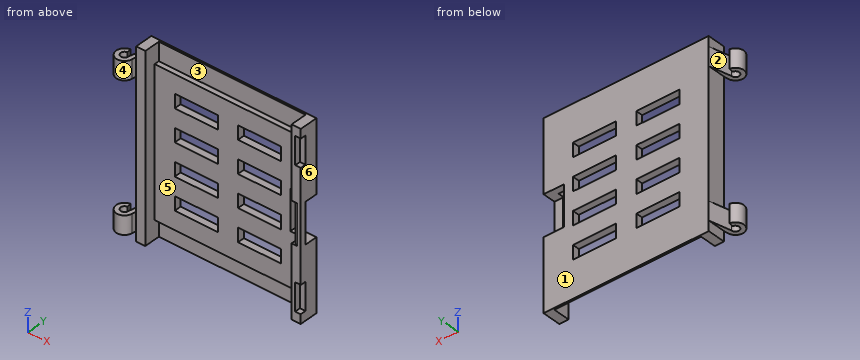
from build123d import *

# Parameters (mm, degrees)
SKETCH1_W           = 3.175
SKETCH1_H           = 1.27
SKETCH1_H_2         = 1.9685
BOSS_EXTRUDE1_DEPTH = 31.75
SKETCH1_4_W         = 3.175
SKETCH1_4_H         = 1.27
CUT_EXTRUDE1_DEPTH  = 6.985
SKETCH2_W           = 3.429
SKETCH2_H           = 10.222992
SKETCH2_W_2         = 13.9065
SKETCH2_W_3         = 6.35
CUT_EXTRUDE2_DEPTH  = 19.05
SKETCH4_W           = 14.9225
SKETCH4_H           = 4.7625
CUT_EXTRUDE4_DEPTH  = 3.38125
CUT_EXTRUDE7_DEPTH  = 6.985
SKETCH9_W           = 50.8
SKETCH9_H           = 1.74625
CUT_EXTRUDE8_DEPTH  = 6.35
SKETCH10_W          = 9.525
SKETCH10_H          = 1.905
CUT_EXTRUDE9_DEPTH  = 1.905
SKETCH11_W          = 3.175
SKETCH11_H          = 0.1905
CUT_EXTRUDE10_DEPTH = 64.5
FILLET2_R           = 0.127


with BuildPart() as part:
    # Sketch1 → Boss-Extrude1 (new body, symmetric)
    with BuildSketch(Plane.XY):
        Polygon((-28.575, 6.35), (-28.575, 0), (-25.4, 0), (-25.4, 3.96875), (21.59, 3.96875), (21.59, 6.35), align=None)
        with BuildLine():
            Line((-28.719147778, -1.313425633), (-28.575, 0))
            Line((-28.575, 0), (-28.575, 6.35))
            Line((-28.575, 6.35), (-30.257496, -0.999998))
            ThreePointArc((-30.257496, -0.999998), (-32.447762596, -1.986950865), (-31.736171426, 0.307603934))
            Line((-31.736171426, 0.307603934), (-31.926464573, 1.851416204))
            ThreePointArc((-31.926464573, 1.851416204), (-33.592921231, -3.045007588), (-28.719147778, -1.313425633))
        make_face()
        Polygon((28.575, 6.35), (21.59, 6.35), (21.59, 3.96875), (25.4, 3.96875), (25.4, 3.2385), (28.575, 3.2385), align=None)
        with Locations((26.9875, 2.6035)):
            Rectangle(SKETCH1_W, SKETCH1_H)
        with Locations((26.9875, 0.98425)):
            Rectangle(SKETCH1_W, SKETCH1_H_2)
    extrude(amount=BOSS_EXTRUDE1_DEPTH, both=True)

    # Sketch1_4 → Cut-Extrude1 (cut, symmetric)
    with BuildSketch(Plane.XY):
        with Locations((26.9875, 2.6035)):
            Rectangle(SKETCH1_4_W, SKETCH1_4_H)
        Polygon((28.575, 6.35), (21.59, 6.35), (21.59, 3.96875), (25.4, 3.96875), (25.4, 3.2385), (28.575, 3.2385), align=None)
    extrude(amount=CUT_EXTRUDE1_DEPTH, both=True, mode=Mode.SUBTRACT)

    # Sketch2 → Cut-Extrude2 (cut)
    with BuildSketch(Plane(origin=(-28.575, 9.604995709, 0), x_dir=(0, 0, 1), z_dir=(-1, 0, 0))):
        with Locations((-30.0355, -8.366491709)):
            Rectangle(SKETCH2_W, SKETCH2_H)
        with Locations((-15.01775, -8.366491709)):
            Rectangle(SKETCH2_W_2, SKETCH2_H)
        with Locations((-4.8895, -8.366491709)):
            Rectangle(SKETCH2_W_3, SKETCH2_H)
        with Locations((4.8895, -8.366491709)):
            Rectangle(SKETCH2_W_3, SKETCH2_H)
        with Locations((15.01775, -8.366491709)):
            Rectangle(SKETCH2_W_2, SKETCH2_H)
        with Locations((30.0355, -8.366491709)):
            Rectangle(SKETCH2_W, SKETCH2_H)
        with Locations((0, -8.366491709)):
            Rectangle(SKETCH2_W, SKETCH2_H)
    extrude(amount=CUT_EXTRUDE2_DEPTH, mode=Mode.SUBTRACT)

    # Sketch4 → Cut-Extrude4 (cut, through all)
    with BuildSketch(Plane.XZ.offset(-3.96875)):
        with Locations((-10.95375, 16.66875)):
            Rectangle(SKETCH4_W, SKETCH4_H)
        with Locations((10.95375, 16.66875)):
            Rectangle(SKETCH4_W, SKETCH4_H)
        with Locations((-10.95375, 5.55625)):
            Rectangle(SKETCH4_W, SKETCH4_H)
        with Locations((10.95375, 5.55625)):
            Rectangle(SKETCH4_W, SKETCH4_H)
        with Locations((-10.95375, -5.55625)):
            Rectangle(SKETCH4_W, SKETCH4_H)
        with Locations((10.95375, -5.55625)):
            Rectangle(SKETCH4_W, SKETCH4_H)
        with Locations((-10.95375, -16.66875)):
            Rectangle(SKETCH4_W, SKETCH4_H)
        with Locations((10.95375, -16.66875)):
            Rectangle(SKETCH4_W, SKETCH4_H)
    extrude(amount=-CUT_EXTRUDE4_DEPTH, mode=Mode.SUBTRACT)

    # Sketch8 → Cut-Extrude7 (cut, symmetric)
    with BuildSketch(Plane.XY):
        with BuildLine():
            ThreePointArc((27.432, 0), (26.172949082, 0.772949082), (25.4, 2.032))
            ThreePointArc((25.4, 2.032), (25.995159021, 0.595159021), (27.432, 0))
        make_face()
        with BuildLine():
            ThreePointArc((25.4, 2.032), (25.995159021, 0.595159021), (27.432, 0))
            Line((27.432, 0), (25.4, 0))
            Line((25.4, 0), (25.4, 2.032))
        make_face()
    extrude(amount=CUT_EXTRUDE7_DEPTH, both=True, mode=Mode.SUBTRACT)

    # Sketch9 → Cut-Extrude8 (cut)
    with BuildSketch(Plane.XY.offset(31.75)):
        with Locations((0, 4.841875)):
            Rectangle(SKETCH9_W, SKETCH9_H)
    cut_extrude8 = extrude(amount=-CUT_EXTRUDE8_DEPTH, mode=Mode.SUBTRACT)

    # Mirror1: Cut-Extrude8 across plane
    add(cut_extrude8.mirror(Plane.XY), mode=Mode.SUBTRACT)

    # Sketch10 → Cut-Extrude9 (cut)
    with BuildSketch(Plane(origin=(28.575, 0, 0), x_dir=(0, 0, -1), z_dir=(1, 0, 0))):
        with Locations((23.8125, 0.9525)):
            Rectangle(SKETCH10_W, SKETCH10_H)
        with Locations((-23.8125, 0.9525)):
            Rectangle(SKETCH10_W, SKETCH10_H)
    extrude(amount=-CUT_EXTRUDE9_DEPTH, mode=Mode.SUBTRACT)

    # Sketch11 → Cut-Extrude10 (cut, through all)
    with BuildSketch(Plane.XY.offset(31.75)):
        with Locations((-26.9875, 0.09525)):
            Rectangle(SKETCH11_W, SKETCH11_H)
    extrude(amount=-CUT_EXTRUDE10_DEPTH, mode=Mode.SUBTRACT)

    # Fillet2
    fillet2_edges = [part.edges().sort_by_distance(p)[0] for p in [
        (25.421490589, 1.9685, 0),
    ]]
    fillet(fillet2_edges, radius=FILLET2_R)


solid = part.part
The listing builds one solid part. Answer for the finished solid, in the listing's coordinates (mm). Face numbers are marked on the shaded views. A direction names the side the tool comes from. Coordinates: 2 decimals unless noted, no trailing zeros. Answer in a Markdown table with one row per item.
1) Find section A-A (z = -6). Count the separate pieces of the cut face and the enclosed holes in it, then the cut area to 3 significant figures.
Answers below:
| item | result |
|---|---|
| separate pieces | 4 |
| enclosed holes | 0 |
| area | 65.2 mm^2 |
2) Given pin 1 (1.8 mm diameter, centred on x = -32.5, y = -1, fed in from +Z); pin 2 (1.4 mm diameter, centred on x = 12, y = 4.5, fed in from -Z); pin 3 (1.7 mm diameter, centred on y = 3, z = 20, fed in from -X) (3 decimals), each flat-ended and moving along its own axis, determine where each tip first touches the part or whether it passes through.
Answers below:
| item | result |
|---|---|
| pin 1 | z = 28.32 |
| pin 2 | z = -25.4 |
| pin 3 | x = -28.575 |
3) Determine the mould class of the marked faces 4, 5 and 6 for opening direction X: released by +X, released by -X, zero draft, split by the parting line, or undercut.
Answers below:
| item | result |
|---|---|
| face 4 | split by the parting line |
| face 5 | undercut |
| face 6 | released by +X |
4) Find the intervals of material crossed by probe 1 along X at (y, z) = (6.25, 18) (1 decimal); probe 2 along X at (y, z) = (2.75, 12.5) (3 decimals); probe 3 along X at (y, z) = (5.5, -4) (1 decimal), in increasing order.
Answers below:
| item | result |
|---|---|
| probe 1 | -28.6 to -18.4, -3.5 to 3.5, 18.4 to 28.6 |
| probe 2 | -28.575 to -25.4, 25.4 to 28.575 |
| probe 3 | -28.6 to -18.4, -3.5 to 3.5, 18.4 to 21.6 |
5) Which of the six approach directions +Z, -Z, +X, -X, +Y, -Y give full straight-line access (tool end or side, diameter ignored) to the marked faces 1, 2 and 3?
Answers below:
| item | result |
|---|---|
| face 1 | +Z, -Z, +X, -X, +Y |
| face 2 | +Z, -Z, +Y |
| face 3 | +Z, -Y |
